Part model, mm, in its own coordinate system. A direction names the side the tool comes from. Give positions to 0.01 mm unless a question says otherwise; leave off trailing zeros. Order: outer loops, then holes, each group sorted by start corner. A loop starts at its lowest first (then second) coordinate and runs counter-clockwise, first axis right, second up. Notation, with made-up numbers: M 77.25,-7 L 82.25,-7 A22 ccw 82.25,17 Z; hole C 79,16.5 d5. An arc over 180 degrees is marked long. One line per question, with ' | ' between items.
```python
from build123d import *

# Parameters (mm, degrees)
SKETCH1_W           = 29.5
SKETCH1_H           = 13
BOSS_EXTRUDE1_DEPTH = 5
SKETCH2_W           = 10
SKETCH2_H           = 6
CUT_EXTRUDE1_DEPTH  = 6
FILLET1_R           = 2
FILLET2_R           = 1.5
SKETCH3_OUTSIDE_W   = 38.024
SKETCH3_OUTSIDE_H   = 13.524
SKETCH3_OUTSIDE_W_2 = 20.5
SKETCH3_OUTSIDE_H_2 = 5
CUT_EXTRUDE2_DEPTH  = 2


with BuildPart() as part:
    # Sketch1 → Boss-Extrude1 (new body)
    with BuildSketch(Plane(origin=(0, 0, 0), x_dir=(1, 0, 0), z_dir=(0, 1, 0))):
        Rectangle(SKETCH1_W, SKETCH1_H)
    extrude(amount=BOSS_EXTRUDE1_DEPTH)

    # Sketch2 → Cut-Extrude1 (cut, through all)
    with BuildSketch(Plane(origin=(0, 5, 0), x_dir=(1, 0, 0), z_dir=(0, 1, 0))):
        with Locations((0, -3.5)):
            Rectangle(SKETCH2_W, SKETCH2_H)
    extrude(amount=-CUT_EXTRUDE1_DEPTH, mode=Mode.SUBTRACT)

    # Fillet1
    fillet1_edges = [part.edges().sort_by_distance(p)[0] for p in [
        (-14.75, 2.5, -6.5),
        (14.75, 2.5, -6.5),
    ]]
    fillet(fillet1_edges, radius=FILLET1_R)

    # Fillet2
    fillet2_edges = [part.edges().sort_by_distance(p)[0] for p in [
        (-5, 2.5, 0.5),
        (5, 2.5, 0.5),
    ]]
    fillet(fillet2_edges, radius=FILLET2_R)

    # Sketch3 outside → Cut-Extrude2 (cut)
    with BuildSketch(Plane.XY.offset(6.5)):
        with Locations((0, 2.5)):
            Rectangle(SKETCH3_OUTSIDE_W, SKETCH3_OUTSIDE_H)
        with Locations((0, 2.5)):
            Rectangle(SKETCH3_OUTSIDE_W_2, SKETCH3_OUTSIDE_H_2, mode=Mode.SUBTRACT)
    extrude(amount=-CUT_EXTRUDE2_DEPTH, mode=Mode.SUBTRACT)


solid = part.part
```
1. Slice it at D-D on x = -3. Give the cut face in (y, z), then the cut area to 3 significant figures.
Worked out:
outline: M 0,-6.5 L 5,-6.5 L 5,0.5 L 0,0.5 Z | area: 35.0 mm2
2. Tool access for faces 4 (the flat face through (14.75, 2, 0)), 5 (the flat face through (-13, 3, 4.5)), 6 (the flat face through (12, 3, 4.5)), 7 (the cylindrical face through (-4.57, 2.46, 0.95)), 8 (the flat face through (8, 2, 6.5)): list every direction of +Z, -Z, +X, -X, +Y, -Y with a clear straight run to the whole face (end or side of a thin tool).
Worked out:
face 4: +Z, -Z, +X, +Y, -Y | face 5: +Z, -X, +Y, -Y | face 6: +Z, +X, +Y, -Y | face 7: +Z, +Y, -Y | face 8: +Z, +X, -X, +Y, -Y
3. Slice it at C-C on z = 5.25. Give the cut face in (x, y).
Worked out:
outline: M -10.25,0 L -5,0 L -5,5 L -10.25,5 Z; M 5,0 L 10.25,0 L 10.25,5 L 5,5 Z
4. Probe L1, parallel to X at y = 2.45, z = 5.75; L2, parallel to X at y = 0.4, z = 4.25; L3, parallel to Z at x = 11, y = 0.7. List the from-to ranges inside material, lowest first. Write a range as from..to.
Worked out:
L1: x = -10.25..-5, 5..10.25 | L2: x = -14.75..-5, 5..14.75 | L3: z = -6.5..4.5
5. Drop flat-ended pins along their axis: pin 1 (2 mm diameter, centred on x = -13, y = 2.5, fed in from +Z); pin 2 (0.6 mm diameter, centred on y = 1.5, z = 5, fed in from +X); pin 3 (0.6 mm diameter, centred on y = 3, z = 5.5, fed in from -X). Give the stop position or say it passes through.
Worked out:
pin 1: stops at z = 4.5 | pin 2: stops at x = 10.25 | pin 3: stops at x = -10.25
6. Slice it at A-A on z = 3.25. Give the cut face in (x, y).
Worked out:
outline: M -14.75,0 L -5,0 L -5,5 L -14.75,5 Z; M 5,0 L 14.75,0 L 14.75,5 L 5,5 Z
7. Slice it at B-B on y = 1.45. Give the cut face in (x, z), then the cut area to 3 significant figures.
Worked out:
outline: M -14.75,-4.5 A2 ccw -12.75,-6.5 L 12.75,-6.5 A2 ccw 14.75,-4.5 L 14.75,4.5 L 10.25,4.5 L 10.25,6.5 L 5,6.5 L 5,2 A1.5 cw 3.5,0.5 L -3.5,0.5 A1.5 cw -5,2 L -5,6.5 L -10.25,6.5 L -10.25,4.5 L -14.75,4.5 Z | area: 305 mm2
8. Mould opens along X. For faces 1 (the flat face through (0, 0, -2)), 2 (the flat face through (5, 3, 4)), 3 (the flat face through (-10.25, 2, 6)) say: released by +X, released by -X, zero draft, split by the parting line, or undercut.
Worked out:
face 1: zero draft | face 2: undercut | face 3: released by -X
